Source: CAD feature listing. Evaluate the final solid. Frame: model axes, mm. A direction names the side the tool comes from. Give positions to 0.01 mm unless a question says otherwise; leave off trailing zeros. Loops run counter-clockwise (first coordinate to the right, second up) from the corner with the lowest first, then second, coordinate; pieces in that order, holes last. Notation, with made-up numbers: (54, 24) -> (79, 24) arc R13 ccw to (79, 36) -> close; hole circle Ø7 at (-34, -35.5). An arc over 180 degrees is marked (long way). Put each result on its own line as item: value.
```python
from build123d import *

# Parameters (mm, degrees)
SKETCH1_R           = 2.5
BOSS_EXTRUDE1_DEPTH = 50
SCALE_2_SCALE       = 3
SCALE_3_SCALE       = 6
SCALE_5_SCALE       = 2
SCALE_6_SCALE       = 0.25
SCALE_7_SCALE       = 0.125
SCALE_8_SCALE       = 0.25
SCALE_9_SCALE       = 4
SCALE_10_SCALE      = 4
OTHER_START         = -17.55
OTHER_1_OUTLINE_R   = 5
OTHER_1_DEPTH       = 10


# Read off the part's stored shape, not the designer's step: 孔1
with BuildPart() as part:
    # Sketch1 → Boss-Extrude1 (new body)
    with BuildSketch(Plane.XY):
        with BuildLine():
            Line((2.839339828, 3.9), (5.5, 6.560660172))
            Line((5.5, 6.560660172), (5.5, 8.2))
            Line((5.5, 8.2), (3.1, 8.2))
            Line((3.1, 8.2), (3.1, 9.5))
            Line((3.1, 9.5), (3.6, 9.5))
            Line((3.6, 9.5), (3.6, 10))
            Line((3.6, 10), (8.5, 10))
            ThreePointArc((8.5, 10), (9.560660172, 9.560660172), (10, 8.5))
            Line((10, 8.5), (10, 3.6))
            Line((10, 3.6), (9.5, 3.6))
            Line((9.5, 3.6), (9.5, 3.1))
            Line((9.5, 3.1), (8.2, 3.1))
            Line((8.2, 3.1), (8.2, 5.5))
            Line((8.2, 5.5), (6.560660172, 5.5))
            Line((6.560660172, 5.5), (3.9, 2.839339828))
            Line((3.9, 2.839339828), (3.9, -2.839339828))
            Line((3.9, -2.839339828), (6.560660172, -5.5))
            Line((6.560660172, -5.5), (8.2, -5.5))
            Line((8.2, -5.5), (8.2, -3.1))
            Line((8.2, -3.1), (9.5, -3.1))
            Line((9.5, -3.1), (9.5, -3.6))
            Line((9.5, -3.6), (10, -3.6))
            Line((10, -3.6), (10, -8.5))
            ThreePointArc((10, -8.5), (9.560660172, -9.560660172), (8.5, -10))
            Line((8.5, -10), (3.6, -10))
            Line((3.6, -10), (3.6, -9.5))
            Line((3.6, -9.5), (3.1, -9.5))
            Line((3.1, -9.5), (3.1, -8.2))
            Line((3.1, -8.2), (5.5, -8.2))
            Line((5.5, -8.2), (5.5, -6.560660172))
            Line((5.5, -6.560660172), (2.839339828, -3.9))
            Line((2.839339828, -3.9), (-2.839339828, -3.9))
            Line((-2.839339828, -3.9), (-5.5, -6.560660172))
            Line((-5.5, -6.560660172), (-5.5, -8.2))
            Line((-5.5, -8.2), (-3.1, -8.2))
            Line((-3.1, -8.2), (-3.1, -9.5))
            Line((-3.1, -9.5), (-3.6, -9.5))
            Line((-3.6, -9.5), (-3.6, -10))
            Line((-3.6, -10), (-8.5, -10))
            ThreePointArc((-8.5, -10), (-9.560660172, -9.560660172), (-10, -8.5))
            Line((-10, -8.5), (-10, -3.6))
            Line((-10, -3.6), (-9.5, -3.6))
            Line((-9.5, -3.6), (-9.5, -3.1))
            Line((-9.5, -3.1), (-8.2, -3.1))
            Line((-8.2, -3.1), (-8.2, -5.5))
            Line((-8.2, -5.5), (-6.560660172, -5.5))
            Line((-6.560660172, -5.5), (-3.9, -2.839339828))
            Line((-3.9, -2.839339828), (-3.9, 2.839339828))
            Line((-3.9, 2.839339828), (-6.560660172, 5.5))
            Line((-6.560660172, 5.5), (-8.2, 5.5))
            Line((-8.2, 5.5), (-8.2, 3.1))
            Line((-8.2, 3.1), (-9.5, 3.1))
            Line((-9.5, 3.1), (-9.5, 3.6))
            Line((-9.5, 3.6), (-10, 3.6))
            Line((-10, 3.6), (-10, 8.5))
            ThreePointArc((-10, 8.5), (-9.560660172, 9.560660172), (-8.5, 10))
            Line((-8.5, 10), (-3.6, 10))
            Line((-3.6, 10), (-3.6, 9.5))
            Line((-3.6, 9.5), (-3.1, 9.5))
            Line((-3.1, 9.5), (-3.1, 8.2))
            Line((-3.1, 8.2), (-5.5, 8.2))
            Line((-5.5, 8.2), (-5.5, 6.560660172))
            Line((-5.5, 6.560660172), (-2.839339828, 3.9))
            Line((-2.839339828, 3.9), (2.839339828, 3.9))
        make_face()
        with Locations((0, 0.235847297)):
            Circle(SKETCH1_R, mode=Mode.SUBTRACT)
    extrude(amount=BOSS_EXTRUDE1_DEPTH)


with BuildPart() as part_1:
    # 缩放比例2: scaled about (0, -0.027095247, 25)
    add(part.part.scale(SCALE_2_SCALE).moved(Location((0, 0.054190494, -50))))


with BuildPart() as part_2:
    # 缩放比例3: scaled about (0, -0.027095247, 25)
    add(part_1.part.scale(SCALE_3_SCALE).moved(Location((0, 0.135476235, -125))))


with BuildPart() as part_3:
    # 缩放比例5: scaled about (0, -0.027095249, 25)
    add(part_2.part.scale(SCALE_5_SCALE).moved(Location((0, 0.027095249, -25))))


with BuildPart() as part_4:
    # 缩放比例6: scaled about (0, -0.027095249, 25)
    add(part_3.part.scale(SCALE_6_SCALE).moved(Location((0, -0.020321437, 18.75))))


with BuildPart() as part_5:
    # 缩放比例7: scaled about (0, -0.027095249, 25)
    add(part_4.part.scale(SCALE_7_SCALE).moved(Location((0, -0.023708343, 21.875))))


with BuildPart() as part_6:
    # 缩放比例8: scaled about (0, -0.027095249, 25)
    add(part_5.part.scale(SCALE_8_SCALE).moved(Location((0, -0.020321437, 18.75))))


with BuildPart() as part_7:
    # 缩放比例9: scaled about (0, -0.027095249, 25)
    add(part_6.part.scale(SCALE_9_SCALE).moved(Location((0, 0.081285747, -75))))


with BuildPart() as part_8:
    # 缩放比例10: scaled about (0, -0.027095249, 25)
    add(part_7.part.scale(SCALE_10_SCALE).moved(Location((0, 0.081285747, -75))))

    # 孔1 outline → 孔1 (cut)
    with BuildSketch(Plane.YZ.offset(OTHER_START)):
        with Locations((7.344833538, 1.297306883)):
            Circle(OTHER_1_OUTLINE_R)
    extrude(amount=OTHER_1_DEPTH, mode=Mode.SUBTRACT)


solid = part_8.part
```
(1) Section B-B on y = 20. Return loops of the section in (x, z).
Calculated:
outline: (-45, -87.5) -> (-36.9, -87.5) -> (-36.9, 137.5) -> (-45, 137.5) -> close; (-24.68, -87.5) -> (-15.13, -87.5) -> (-15.13, 137.5) -> (-24.68, 137.5) -> close; (15.13, -87.5) -> (24.68, -87.5) -> (24.68, 137.5) -> (15.13, 137.5) -> close; (36.9, -87.5) -> (45, -87.5) -> (45, 137.5) -> (36.9, 137.5) -> close
(2) Draft query along X for faces 4 (the flat face through (17.55, 0, 23)), 5 (the flat face through (-36.9, -19, 23)), 6 (the flat face through (40, -13.855, 23)). Return one class per face: released by +X, released by -X, zero draft, split by the parting line, or undercut.
Calculated:
face 4: released by +X
face 5: undercut
face 6: zero draft
(3) Section D-D on x = 21. Return loops of the section in (y, z).
Calculated:
outline: (-44.91, -87.5) -> (-36.81, -87.5) -> (-36.81, 137.5) -> (-44.91, 137.5) -> close; (-25.68, -87.5) -> (-16.13, -87.5) -> (-16.13, 137.5) -> (-25.68, 137.5) -> close; (16.32, -87.5) -> (25.87, -87.5) -> (25.87, 137.5) -> (16.32, 137.5) -> close; (36.99, -87.5) -> (45.09, -87.5) -> (45.09, 137.5) -> (36.99, 137.5) -> close
(4) Line query: probe 1 along Y at (x, z) = (-39, -49.5); probe 2 along X at (y, z) = (-35, 21); probe 3 along X at (y, z) = (-38, -14.5). Output: solid intervals per line, ascending. Write a range as from..to.
Calculated:
probe 1: y = -44.86..-13.86, 14.04..45.05
probe 2: x = -45..-24.75, 24.75..45
probe 3: x = -45..-13.95, 13.95..45
(5) Section A-A on x = -33. Return loops of the section in (y, z).
Calculated:
outline: (-44.91, -87.5) -> (-24.66, -87.5) -> (-24.66, 137.5) -> (-44.91, 137.5) -> close; (24.84, -87.5) -> (45.09, -87.5) -> (45.09, 137.5) -> (24.84, 137.5) -> close
(6) Section C-C on x = 0. Return loops of the section in (y, z), then the cut area to 4 significant figures.
Calculated:
outline: (-17.46, -87.5) -> (-10.09, -87.5) -> (-10.09, 137.5) -> (-17.46, 137.5) -> close; (12.41, -87.5) -> (17.64, -87.5) -> (17.64, 137.5) -> (12.41, 137.5) -> close
area: 2,835 mm²
(7) First-contact query: P1, Ø1.8, axis at y = 44, z = 38.5, coming from the -X side; P2, Ø1.1, axis at x = -15.5, z = -8, coming from the -Y side; P3, Ø1.1, axis at y = 15.5, z = 59, coming from the +X side. Flat tips, straight axial feed; report the tip coordinate or a pass-through.
Calculated:
P1: stops at x = -43.04
P2: stops at y = -42.66
P3: stops at x = 42.75
(8) Reachability of faces 1 (the flat face through (-23.45, 18.77, 23.43)), 2 (the flat face through (0, 17.645, 23)), 3 (the flat face through (-40, -13.855, 23)) from +Z, -Z, +X, -X, +Y, -Y: full face, straight path, thin tool, end or side. Return the list, or none.
Calculated:
face 1: +Z, -Z
face 2: +Z, -Z, +Y
face 3: +Z, -Z, -X
